```python
from build123d import *

# Parameters (mm, degrees)
BOSS_EXTRUDE1_DEPTH       = 64.5
SKETCH3_W                 = 62
SKETCH3_H                 = 121
BOSS_EXTRUDE3_DEPTH       = 4.5
SKETCH6_W                 = 40
SKETCH6_H                 = 98
CUT_EXTRUDE3_DEPTH        = 7
SKETCH5_W                 = 57.24
SKETCH5_H                 = 111
CUT_EXTRUDE2_DEPTH        = 1.23
CUT_EXTRUDE1_DEPTH        = 111
CUT_EXTRUDE4_REACH        = 90.677
SKETCH7_R                 = 1.925
SKETCH7_RX                = 2.5
SKETCH7_RY                = 1.85
F_1_0MM_DOWEL_HOLE1_D     = 3.5
F_1_0MM_DOWEL_HOLE1_DEPTH = 7
SKETCH10_W                = 20
SKETCH10_H                = 13
CUT_EXTRUDE5_DEPTH        = 10
SKETCH11_W                = 11
SKETCH11_H                = 43
CUT_EXTRUDE6_DEPTH        = 2.5
SKETCH12_W                = 2
SKETCH12_H                = 8.260777535
CUT_EXTRUDE7_DEPTH        = 153.121661837


with BuildPart() as part:
    # Sketch1 → Boss-Extrude1 (new, symmetric)
    with BuildSketch(Plane.XY):
        Polygon((0, 0), (70, 0), (10, 40), (0, 40), align=None)
    extrude(amount=BOSS_EXTRUDE1_DEPTH, both=True)

    # Sketch3 → Boss-Extrude3 (add)
    with BuildSketch(Plane.XZ):
        with Locations((35, 0)):
            Rectangle(SKETCH3_W, SKETCH3_H)
    extrude(amount=BOSS_EXTRUDE3_DEPTH)

    # Sketch6 → Cut-Extrude3 (cut)
    with BuildSketch(Plane(origin=(21.538461538, 32.307692308, 0), x_dir=(0.8320502943378438, -0.5547001962252291, 0), z_dir=(0.5547001962252291, 0.8320502943378438, 0))):
        with Locations((23.632495094, 2.5)):
            Rectangle(SKETCH6_W, SKETCH6_H)
    extrude(amount=-CUT_EXTRUDE3_DEPTH, mode=Mode.SUBTRACT)

    # Sketch5 → Cut-Extrude2 (cut)
    with BuildSketch(Plane.XZ.offset(4.5)):
        with Locations((35.18, 0)):
            Rectangle(SKETCH5_W, SKETCH5_H)
    extrude(amount=-CUT_EXTRUDE2_DEPTH, mode=Mode.SUBTRACT)

    # Sketch4 → Cut-Extrude1 (cut)
    with BuildSketch(Plane.XY.offset(55.5)):
        Polygon((63.780493494, -4.266615306), (6.558549313, 33.881347482), (6.558549313, -4.5), (63.780493494, -4.5), align=None)
    extrude(amount=-CUT_EXTRUDE1_DEPTH, mode=Mode.SUBTRACT)

    # Sketch7 → Cut-Extrude4 (cut, up to next)
    with BuildSketch(Plane(origin=(21.538461538, 32.307692308, 0), x_dir=(0.8320502943378438, -0.5547001962252291, 0), z_dir=(0.5547001962252291, 0.8320502943378438, 0)), mode=Mode.PRIVATE) as cut_extrude4_sk1:
        with Locations(Location((29.882495094, -51, 0), (0, 0, 180))):
            Circle(SKETCH7_R)
    cut_extrude4_tool1 = extrude(cut_extrude4_sk1.sketch, amount=-CUT_EXTRUDE4_REACH, mode=Mode.PRIVATE) & part.part
    # Sketch7 → Cut-Extrude4 (cut, up to next)
    with BuildSketch(Plane(origin=(21.538461538, 32.307692308, 0), x_dir=(0.8320502943378438, -0.5547001962252291, 0), z_dir=(0.5547001962252291, 0.8320502943378438, 0)), mode=Mode.PRIVATE) as cut_extrude4_sk2:
        with Locations((17.382495094, -51)):
            Ellipse(SKETCH7_RX, SKETCH7_RY)
    cut_extrude4_tool2 = extrude(cut_extrude4_sk2.sketch, amount=-CUT_EXTRUDE4_REACH, mode=Mode.PRIVATE) & part.part
    add(cut_extrude4_tool1.solids().sort_by_distance((46.4022, 15.731866, 51))[0], mode=Mode.SUBTRACT)
    add(cut_extrude4_tool2.solids().sort_by_distance((36.001572, 22.665619, 51))[0], mode=Mode.SUBTRACT)

    # Ø1.0mm Dowel Hole1
    with Locations(Plane(origin=(21.538461538, 32.307692308, 0), x_dir=(0.8320502943378438, -0.5547001962252291, 0), z_dir=(0.5547001962252291, 0.8320502943378438, 0))):
        with Locations((-3.867504906, -44), (-3.867504906, 49), (51.132495094, 49), (51.132495094, -44)):
            Hole(F_1_0MM_DOWEL_HOLE1_D / 2, depth=F_1_0MM_DOWEL_HOLE1_DEPTH)

    # Sketch10 → Cut-Extrude5 (cut)
    with BuildSketch(Plane.ZY):
        with Locations((45.5, 9.5)):
            Rectangle(SKETCH10_W, SKETCH10_H)
    extrude(amount=-CUT_EXTRUDE5_DEPTH, mode=Mode.SUBTRACT)

    # Sketch11 → Cut-Extrude6 (cut)
    with BuildSketch(Plane(origin=(17.655560165, 26.483340247, 0), x_dir=(0.8320502943378436, -0.5547001962252294, 0), z_dir=(-0.5547001962252293, -0.8320502943378435, 0))):
        with Locations((-1.867504906, 17.5)):
            Rectangle(SKETCH11_W, SKETCH11_H)
    extrude(amount=-CUT_EXTRUDE6_DEPTH, mode=Mode.SUBTRACT)

    # Sketch12 → Cut-Extrude7 (cut, through all)
    with BuildSketch(Plane.XY.offset(64.5)):
        with Locations((70, 0.079119359)):
            Rectangle(SKETCH12_W, SKETCH12_H)
    extrude(amount=-CUT_EXTRUDE7_DEPTH, mode=Mode.SUBTRACT)


solid = part.part
```
Read the model definition and answer for the solid it produces. Units are mm, in the model's axes. A direction names the side the tool comes from. Give positions to 0.01 mm unless a question says otherwise; leave off trailing zeros. Order: outer loops, then holes, each group sorted by start corner. A loop starts at its lowest first (then second) coordinate and runs counter-clockwise, first axis right, second up.
(1) Find section C-C (z = 28). Give the vertices of the cut face in (x, y), plus the area to 3 significant figures.
(2) Find section A-A (z = -27). Give the vertices of the cut face in (x, y), plus the area to 3 significant figures.
(3) For faces 4 (the flat face through (23.1, 28.1, -1.8)), 5 (the flat face through (3, 3, 45)), 6 (the flat face through (17, 29, 39)), 7 (the flat face through (66, -2, -1)), 8 (the flat face through (4, -2, -1)), determine the directions among +Z, -Z, +X, -X, +Y, -Y from which every point of the face is accessible in a straight line to the end or side of a thin tool.
(4) Given pin 1 (2 mm diameter, centred on x = 54, z = 4.5, fed in from +Y); pin 2 (1.3 mm diameter, centred on x = 47.5, y = -3, fed in from -Z); pin 3 (2 mm diameter, centred on y = -3, z = -7.5, fed in from +X), each flat-ended and moving along its own axis, determine where each tip first touches the part or whether it passes through.
(5) Straight lines are drawn through the part: L1, parallel to Z at x = 19.5, y = 17; L2, parallel to Z at x = 22.5, y = -1.5; L3, parallel to X at y = 12, z = -17.5. For each, find the intervals that lie inside material, in ascending order.
(6) For a pull along Z with two mould halves and no side action, classify faces 1 (the flat face through (35, -2, 60.5)), 2 (the cylindrical face through (61.44, 1.44, 45.55)), 3 (the flat face through (20.2, 33.2, 0.9)) as released by +Z, released by -Z, zero draft, split by the parting line, or undercut.
(7) Find section B-B (x = 52). Give the vertices of the cut face in (y, z).
(8) Find section D-D (y = 6.5). Give the vertices of the cut face in (x, z), plus the area to 3 significant figures.
Result sheet:
1. outline: (0, 0) - (4, 0) - (4, -4.5) - (6.56, -4.5) - (6.56, 33.88) - (11.53, 30.57) - (12.91, 32.65) - (22.06, 26.55) - (24.56, 30.29) - (10, 40) - (0, 40) - close; (53.96, 2.28) - (62.29, -3.27) - (63.8, -3.27) - (63.8, -4.5) - (66, -4.5) - (66, 0) - (69, 0) - (69, 0.67) - (57.84, 8.1) - close
1. area: 466 mm2
2. outline: (0, 0) - (4, 0) - (4, -4.5) - (6.56, -4.5) - (6.56, 33.88) - (20.68, 24.47) - (24.56, 30.29) - (10, 40) - (0, 40) - close; (53.96, 2.28) - (62.29, -3.27) - (63.8, -3.27) - (63.8, -4.5) - (66, -4.5) - (66, 0) - (69, 0) - (69, 0.67) - (57.84, 8.1) - close
2. area: 493 mm2
3. face 4: +X, -Y
3. face 5: -X
3. face 6: -Y
3. face 7: +Z, -Z, +X, -Y
3. face 8: +Z, -Z, -X, -Y
4. pin 1: stops at y = 3.84
4. pin 2: stops at z = -60.5
4. pin 3: stops at x = 66
5. L1: z = -64.5 to -55.5, 55.5 to 64.5
5. L2: z = -60.5 to -55.5, 55.5 to 60.5
5. L3: x = 0 to 6.56
6. face 1: released by +Z
6. face 2: undercut
6. face 3: zero draft
7. outline: (-4.5, -60.5) - (0, -60.5) - (0, -64.5) - (12, -64.5) - (12, -51.5) - (3.59, -51.5) - (3.59, -55.5) - (-4.5, -55.5) - close; (-4.5, 55.5) - (3.59, 55.5) - (3.59, 46.5) - (12, 46.5) - (12, 64.5) - (0, 64.5) - (0, 60.5) - (-4.5, 60.5) - close
8. outline: (0, -64.5) - (60.25, -64.5) - (60.25, 64.5) - (0, 64.5) - (0, 55.5) - (47.63, 55.5) - (47.63, 46.5) - (56.77, 46.5) - (56.77, -51.5) - (47.63, -51.5) - (47.63, -55.5) - (6.56, -55.5) - (6.56, 35.5) - (0, 35.5) - close
8. area: 2,190 mm2
